from build123d import *

# Parameters (mm, degrees)
BOSS_EXTRUDE1_DEPTH = 3


with BuildPart() as part:
    # Sketch1 → Boss-Extrude1 (new body)
    with BuildSketch(Plane.XY):
        with BuildLine():
            Line((-28, 14.725), (-28, -14.725))
            Line((-28, -14.725), (-25.5, -14.725))
            Line((-25.5, -14.725), (-25.5, -17.725))
            Line((-25.5, -17.725), (-19.5, -17.725))
            Line((-19.5, -17.725), (-19.5, -14.725))
            Line((-19.5, -14.725), (-17.5, -14.725))
            ThreePointArc((-17.5, -14.725), (0, 7.78192388), (17.5, -14.725))
            Line((17.5, -14.725), (19.5, -14.725))
            Line((19.5, -14.725), (19.5, -17.725))
            Line((19.5, -17.725), (25.5, -17.725))
            Line((25.5, -17.725), (25.5, -14.725))
            Line((25.5, -14.725), (28, -14.725))
            Line((28, -14.725), (28, 14.725))
            Line((28, 14.725), (25.5, 14.725))
            Line((25.5, 14.725), (25.5, 17.725))
            Line((25.5, 17.725), (19.5, 17.725))
            Line((19.5, 17.725), (19.5, 14.725))
            Line((19.5, 14.725), (-19.5, 14.725))
            Line((-19.5, 14.725), (-19.5, 17.725))
            Line((-19.5, 17.725), (-25.5, 17.725))
            Line((-25.5, 17.725), (-25.5, 14.725))
            Line((-25.5, 14.725), (-28, 14.725))
        make_face()
    extrude(amount=BOSS_EXTRUDE1_DEPTH)


solid = part.part
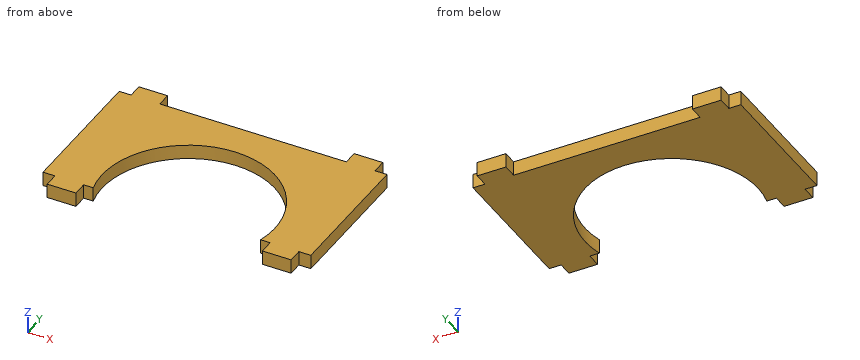
The listing builds one solid part. Answer for the finished solid, in the listing's coordinates (mm). Give positions to 0.01 mm unless a question says otherwise; leave off trailing zeros. Order: outer loops, then holes, each group sorted by start corner. A loop starts at its lowest first (then second) coordinate and runs counter-clockwise, first axis right, second up. Notation, with made-up numbers: (64, 39.25) - (121, 39.25) arc R23 cw to (121, 58.25) - close; hole circle Ø4 at (5, 14.5). An arc over 180 degrees is marked (long way). Answer as CSV lines item,"result".
Q1. Straight lines are drawn through the part: L1, parallel to X at y = -10.5, z = 1.45; L2, parallel to X at y = -16, z = 2.1; L3, parallel to Y at x = 10, z = 1 (3 decimals). For each, find the intervals that lie inside material, in ascending order.
Answer key:
L1,"x = -28 to -18.06, 18.06 to 28"
L2,"x = -25.5 to -19.5, 19.5 to 25.5"
L3,"y = 4.76 to 14.725"
Q2. A cutting plane is placed at A-A, the plane y = 0. Determine the outline of the cut face in (x, z), and give its area (3 significant figures).
Answer key:
outline,"(-28, 0) - (-14.85, 0) - (-14.85, 3) - (-28, 3) - close; (14.85, 0) - (28, 0) - (28, 3) - (14.85, 3) - close"
area,"78.9 mm^2"
Q3. A cutting plane is placed at D-D, the plane x = 14. Determine the outline of the cut face in (y, z) (3 decimals).
Answer key:
outline,"(1.129, 0) - (14.725, 0) - (14.725, 3) - (1.129, 3) - close"
Q4. A cutting plane is placed at B-B, the plane z = 2. Determine the outline of the cut face in (x, y) (3 decimals).
Answer key:
outline,"(-28, -14.725) - (-25.5, -14.725) - (-25.5, -17.725) - (-19.5, -17.725) - (-19.5, -14.725) - (-17.5, -14.725) arc R18.057 cw (long way) to (17.5, -14.725) - (19.5, -14.725) - (19.5, -17.725) - (25.5, -17.725) - (25.5, -14.725) - (28, -14.725) - (28, 14.725) - (25.5, 14.725) - (25.5, 17.725) - (19.5, 17.725) - (19.5, 14.725) - (-19.5, 14.725) - (-19.5, 17.725) - (-25.5, 17.725) - (-25.5, 14.725) - (-28, 14.725) - close"
Q5. A cutting plane is placed at C-C, the plane x = 0. Determine the outline of the cut face in (y, z) (3 decimals), and give its area (3 significant figures).
Answer key:
outline,"(7.782, 0) - (14.725, 0) - (14.725, 3) - (7.782, 3) - close"
area,"20.8 mm^2"
Q6. Each of these flat-tipped pins is pushed along its axis until it touches: pin 1 Ø0.8 at (x, z) = (-26.5, 2) entering from -Y (3 decimals); pin 2 Ø0.9 at (y, z) = (16, 2) entering from +X; pin 3 Ø0.9 at (y, z) = (16, 1) entering from -X; pin 4 Ø2 at (x, y) = (-11, 1.5) entering from -Z (3 decimals). Where does it stop, or does it pass through?
Answer key:
pin 1,"stops at y = -14.725"
pin 2,"stops at x = 25.5"
pin 3,"stops at x = -25.5"
pin 4,"passes through"
